from build123d import *

# Parameters (mm, degrees)
SKETCH1_W           = 20
SKETCH1_H           = 5
BOSS_EXTRUDE1_DEPTH = 2
SKETCH2_R           = 1.1
CUT_EXTRUDE1_DEPTH  = 2
FILLET1_R           = 2.5


with BuildPart() as part:
    # Sketch1 → Boss-Extrude1 (new body)
    with BuildSketch(Plane(origin=(0, 0, 0), x_dir=(1, 0, 0), z_dir=(0, 1, 0))):
        Rectangle(SKETCH1_W, SKETCH1_H)
    extrude(amount=BOSS_EXTRUDE1_DEPTH)

    # Sketch2 → Cut-Extrude1 (cut)
    with BuildSketch(Plane(origin=(0, 2, 0), x_dir=(1, 0, 0), z_dir=(0, 1, 0))):
        with Locations(Location((7.5, 0, 0), (0, 0, 270))):
            Circle(SKETCH2_R)
    extrude(amount=-CUT_EXTRUDE1_DEPTH, mode=Mode.SUBTRACT)

    # Fillet1
    fillet1_edges = [part.edges().sort_by_distance(p)[0] for p in [
        (10, 1, 2.5),
        (10, 1, -2.5),
    ]]
    fillet(fillet1_edges, radius=FILLET1_R - 0.0001)  # a hair under: the kernel refuses the full size


solid = part.part
Geometry check sheet. Reference: the model listing, model coordinates, mm. Round coordinates to 2 decimals unless told otherwise and drop trailing zeros. Loops run counter-clockwise (first coordinate to the right, second up) from the corner with the lowest first, then second, coordinate; pieces in that order, holes last. Notation, with made-up numbers: (-20.75, 20) -> (13.25, 20) arc R13 ccw to (13.25, 29) -> close; hole circle Ø1 at (38, 73.25). An arc over 180 degrees is marked (long way). Answer as a JSON object with one key per item and string values. Group by question number.
Item 1: Cross-section at B-B, the plane x = 7. Record the cut outline in (y, z).
Item 2: Release check for a two-part mould opening along X. For faces 1 (the face through (-1, 1, -2.5)), 2 (the face through (7.5, 1, -1.1)), 3 (the face through (-10, 1, 0)) record: pulls with the +X half, pulls with the -X half, needs draft (parallel to the pull), parting line crosses it, or undercut.
Item 3: Cross-section at C-C, the plane z = -0.35. Record the cut outline in (x, y), plus the area to 3 significant figures.
Item 4: Depth check by flat-ended pin: pin 1 Ø3 at (x, z) = (7.5, 0) entering from +Y. Enter the tip coordinate at first touch or a pass-through.
Item 5: Cross-section at D-D, the plane z = -1.8. Record the cut outline in (x, y) (3 decimals).
Item 6: Thickness scan on line 1 along X through (y, z) = (1.1, 0); line 2 along Z through (x, y) = (6.5, 0.15); line 3 along X through (y, z) = (0.9, 0.85). Record the ranges inside material, lowest first.
Determined:
{
 "1": {"outline": "(0, -2.5) -> (2, -2.5) -> (2, -0.98) -> (0, -0.98) -> close; (0, 0.98) -> (2, 0.98) -> (2, 2.5) -> (0, 2.5) -> close"},
 "2": {"face 1": "needs draft", "face 2": "undercut", "face 3": "pulls with the -X half"},
 "3": {"outline": "(-10, 0) -> (6.46, 0) -> (6.46, 2) -> (-10, 2) -> close; (8.54, 0) -> (9.98, 0) -> (9.98, 2) -> (8.54, 2) -> close", "area": "35.8 mm²"},
 "4": {"pin 1": "stops at y = 2"},
 "5": {"outline": "(-10, 0) -> (9.235, 0) -> (9.235, 2) -> (-10, 2) -> close"},
 "6": {"line 1": "x = -10 to 6.4, 8.6 to 10", "line 2": "z = -2.5 to -0.46, 0.46 to 2.5", "line 3": "x = -10 to 6.8, 8.2 to 9.85"}
}
